```python
from build123d import *

# Parameters (mm, degrees)
SKETCH3_W                                     = 76.2
SKETCH3_H                                     = 76.2
BOSS_EXTRUDE3_DEPTH                           = 10
CBORE_FOR_M6_HEX_SOCKET_HEAD_CAP1_D           = 6.6
CBORE_FOR_M6_HEX_SOCKET_HEAD_CAP1_CBORE_D     = 11
CBORE_FOR_M6_HEX_SOCKET_HEAD_CAP1_CBORE_DEPTH = 6
FILLET1_R                                     = 10
SKETCH2_R                                     = 10
BOSS_EXTRUDE4_DEPTH                           = 10
SKETCH9_R                                     = 3.5
CUT_EXTRUDE1_DEPTH                            = 58.473646135
CHAMFER1_SIZE                                 = 1


with BuildPart() as part:
    # Sketch3 → Boss-Extrude3 (new body)
    with BuildSketch(Plane.XY):
        Rectangle(SKETCH3_W, SKETCH3_H)
    extrude(amount=BOSS_EXTRUDE3_DEPTH)

    # CBORE for M6 Hex Socket Head Cap1 (through all)
    with Locations(Plane(origin=(0, 0, 0), x_dir=(-1, 0, 0), z_dir=(0, 0, -1))):
        with Locations((19.05, 19.05), (19.05, -19.05), (-19.05, 19.05), (-19.05, -19.05)):
            CounterBoreHole(CBORE_FOR_M6_HEX_SOCKET_HEAD_CAP1_D / 2, CBORE_FOR_M6_HEX_SOCKET_HEAD_CAP1_CBORE_D / 2, CBORE_FOR_M6_HEX_SOCKET_HEAD_CAP1_CBORE_DEPTH)

    # Fillet1
    fillet1_edges = [part.edges().sort_by_distance(p)[0] for p in [
        (38.1, -38.1, 5),
        (-38.1, -38.1, 5),
        (-38.1, 38.1, 5),
        (38.1, 38.1, 5),
    ]]
    fillet(fillet1_edges, radius=FILLET1_R)

    # Sketch2 → Boss-Extrude4 (add)
    with BuildSketch(Plane(origin=(0, 0, 0), x_dir=(-1, 0, 0), z_dir=(0, 0, -1))):
        Circle(SKETCH2_R)
    extrude(amount=BOSS_EXTRUDE4_DEPTH)

    # Sketch9 → Cut-Extrude1 (cut, through all)
    with BuildSketch(Plane(origin=(0, 0, -10), x_dir=(-1, 0, 0), z_dir=(0, 0, -1))):
        Circle(SKETCH9_R)
    extrude(amount=-CUT_EXTRUDE1_DEPTH, mode=Mode.SUBTRACT)

    # Chamfer1
    chamfer1_edges = [part.edges().sort_by_distance(p)[0] for p in [
        (24.55, -19.05, 0),
        (15.75, -19.05, 10),
        (24.55, 19.05, 0),
        (15.75, 19.05, 10),
        (-13.55, -19.05, 0),
        (-22.35, -19.05, 10),
        (-13.55, 19.05, 0),
        (-22.35, 19.05, 10),
        (0, 38.1, 0),
        (0, 38.1, 10),
        (38.1, 0, 0),
        (0, -38.1, 0),
        (-38.1, 0, 0),
        (-35.171067812, 35.171067812, 0),
        (-35.171067812, -35.171067812, 0),
        (35.171067812, -35.171067812, 0),
        (35.171067812, 35.171067812, 0),
        (38.1, 0, 10),
        (-38.1, 0, 10),
        (0, -38.1, 10),
        (-35.171067812, 35.171067812, 10),
        (-35.171067812, -35.171067812, 10),
        (35.171067812, -35.171067812, 10),
        (35.171067812, 35.171067812, 10),
        (10, 0, -10),
        (3.5, 0, 10),
        (3.5, 0, -10),
    ]]
    chamfer(chamfer1_edges, length=CHAMFER1_SIZE)


solid = part.part
```
Geometry: final body of the model. Coordinates: model frame, mm. A direction names the side the tool comes from. Give positions to 0.01 mm unless a question says otherwise; leave off trailing zeros. Order: outer loops, then holes, each group sorted by start corner. A loop starts at its lowest first (then second) coordinate and runs counter-clockwise, first axis right, second up. Notation, with made-up numbers: M 24.25,82.5 L 52.25,82.5 A26 ccw 52.25,113.5 Z; hole C 7,-15.5 d4. An arc over 180 degrees is marked long. Answer as CSV lines item,"result". Start each with the question number.
1) Cut plane A-A (x = 0). Output: boundary loops of the cut face in (y, z), then the cut area to 3 significant figures.
2) Line query: line 1 (Y direction, x = -19.05, z = 3.2); line 2 (Y direction, x = 19.05, z = 8.45); line 3 (Z direction, x = -25, y = 13). Output: solid intervals per line, ascending. Write a range as from..to.
3) First-contact query: P1, Ø10.5, axis at x = -19.05, y = 19.05, coming from the -Z side; P2, Ø1.5, axis at x = -18, y = -4.5, coming from the -Z side; P3, Ø3.5, axis at x = 20, y = -18, coming from the -Z side; P4, Ø9, axis at x = -19, y = 20.5, coming from the -Z side. Flat tips, straight axial feed; report the tip coordinate or a pass-through.
4) Cut plane C-C (x = 11). Output: boundary loops of the cut face in (y, z), then the cut area to 3 significant figures.
5) Mould query, pull axis X, two halves, no side actions, for faces 3 (the cylindrical face through (35.09, 35.25, 5.06)), 4 (the flat face through (0, -38.1, 5)), 5 (the cylindrical face through (-24.13, -21.16, 3.46)). Classes: +X half, -X half, draft (parallel to the pull), parting line (faces both ways), or undercut.
6) Set-up query: faces 1 (the flat face through (-9, 9, 0)), 2 (the cylindrical face through (-19.77, -22.27, 7.52)). Return all of +Z, -Z, +X, -X, +Y, -Y with unobstructed straight access to the full face (end or side cutting, diameter ignored); none if empty.
7) Cut plane B-B (y = 19.05). State how many separate pieces and enclosed holes the cut face has, then the cut area to 3 significant figures.
Findings below:
1,outline,"M -38.1,1 L -37.1,0 L -10,0 L -10,-9 L -9,-10 L -4.5,-10 L -3.5,-9 L -3.5,9 L -4.5,10 L -37.1,10 L -38.1,9 Z; M 3.5,-9 L 4.5,-10 L 9,-10 L 10,-9 L 10,0 L 37.1,0 L 38.1,1 L 38.1,9 L 37.1,10 L 4.5,10 L 3.5,9 Z"
1,area,"817 mm²"
2,line 1,"y = -38.1..-24.55, -13.55..13.55, 24.55..38.1"
2,line 2,"y = -38.1..-22.35, -15.75..15.75, 22.35..38.1"
2,line 3,"z = 0..10"
3,P1,"stops at z = 6"
3,P2,"stops at z = 0"
3,P3,"passes through"
3,P4,"stops at z = 0.55"
4,outline,"M -38.1,1 L -37.1,0 L 37.1,0 L 38.1,1 L 38.1,9 L 37.1,10 L -37.1,10 L -38.1,9 Z"
4,area,"760 mm²"
5,face 3,"+X half"
5,face 4,"draft"
5,face 5,"undercut"
6,face 1,"-Z"
6,face 2,"+Z, -Z"
7,separate pieces,"3"
7,enclosed holes,"0"
7,area,"571 mm²"
